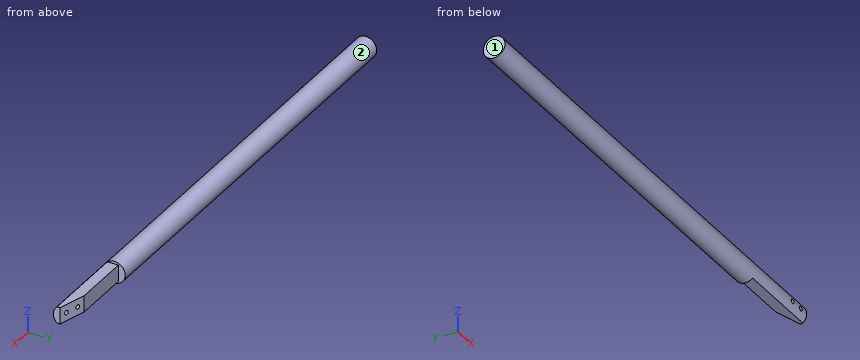
Autodesk Inventor part; units mm, degrees
ref_plane "YZ Plane" through (0, 0, 0) normal (1, 0, 0) x (0, 1, 0)
ref_plane "XZ Plane" through (0, 0, 0) normal (0, 1, 0) x (-1, 0, 0)
ref_plane "XY Plane" through (0, 0, 0) normal (0, 0, 1) x (1, 0, 0)
sketch "Sketch1" plane through (0, 0, 0) normal (1, 0, 0) x (0, 1, 0)
  circle A0 centre (0, 0) radius 6.35
  dimension "d159" = 12.7
extrude "Extrusion1" add sketch "Sketch1" against normal blind 304.8
sketch "Sketch2" plane through (0, 0, 0) normal (1, 0, 0) x (0, 0, -1)
  arc A0 (5.9242, 2.286) -> (-5.9242, 2.286) centre (0, 0) ccw
  circle A1 centre (0, 0) radius 6.35
  line L0 (-5.9242, 2.286) -> (5.9242, 2.286)
  dimension "d111" = 4.064
extrude "Extrusion2" cut sketch "Sketch2" against normal blind 50.8 contours L0 A0
sketch "Sketch5" plane through (0, 2.286, 5.9242) normal (0, 1, 0) x (1, 0, 0)
  line L0 (0, 5.9242) -> (0, 10.7502)
  line L1 (0, 11.8485) -> (0, 0)
  line L2 (0, 10.7502) -> (-50.8, 10.7502)
  line L3 (-50.8, 11.8485) -> (-50.8, 0)
  line L4 (0, 5.9242) -> (0, 1.0982)
  line L5 (0, 1.0982) -> (-50.8, 1.0982)
  line L6 (-50.8, 1.0982) -> (-50.8, -4.826)
  line L7 (-50.8, -4.826) -> (10.2611, -4.826)
  line L8 (10.2611, -4.826) -> (0, 1.0982)
  line L9 (-50.8, 10.7502) -> (-50.8, 16.6745)
  line L10 (-50.8, 16.6745) -> (10.2611, 16.6745)
  line L11 (0, 10.7502) -> (10.2611, 16.6745)
  line L12 (-50.8, 11.8485) -> (0, 11.8485)
  dimension "d20" = 4.826
  dimension "d21" = 4.826
  dimension "d160" = 4.826
extrude "Extrusion3" cut sketch "Sketch5" against normal blind 25.4 contours L2 L3 L12 L1 | L1 L12 L9 L10 L11 | L8 L7 L6 L3 L5
sketch "Sketch18" plane through (-50.8, 2.286, 4.826) normal (0, 0, 1) x (1, 0, 0)
  line L0 (34.4586, 0) -> (50.8, -4.6858)
  line L1 (0, 0) -> (50.8, 0)
  line L2 (34.4586, 0) -> (50.8, 0)
  line L3 (50.8, 0) -> (50.8, -4.6858)
  dimension "d144" = 17
  dimension "d161" = 74
extrude "Extrusion9" cut sketch "Sketch18" against normal blind 25.4
sketch "Sketch19" plane through (-16.3414, 2.286, 4.826) normal (0.2756374, 0.9612617, 0) x (0.9612617, -0.2756374, 0)
  circle A0 centre (12.4695, 4.826) radius 1.5875
  circle A1 centre (4.532, 4.826) radius 1.5875
  line L0 (14.057, 4.826) -> (17, 4.826)
  line L1 (17, 9.652) -> (17, 0)
  line L2 (14.057, 4.826) -> (4.532, 4.826) construction
  dimension "d148" = 3.175
  dimension "d149" = 3.175
  dimension "d151" = 7.9375
  dimension "d162" = 2.943
hole "Hole9" at (-11.985, 1.0368, 0) at (-4.355, -1.1511, 0) direction (-0.2756374, -0.9612617, 0) diameter 2.4867 end through all
equation "\"d160\" = d20"
properties part number "rat_headbarAngled" material "Stainless Steel"
Check sheet for the modelled part. Datum: model origin and axes. Units: mm. Face numbers are marked on the shaded views. Give positions to 0.01 mm unless a question says otherwise; leave off trailing zeros. Order: outer loops, then holes, each group sorted by start corner. A loop starts at its lowest first (then second) coordinate and runs counter-clockwise, first axis right, second up. Notation, with made-up numbers: M 77.5,0 L 86.5,0 A14 ccw 86.5,9 Z; hole C 36,22.5 d10. An arc over 180 degrees is marked long. Answer as CSV lines item,"result". Start each with the question number.
Item 1: Thickness scan on line 1 (X direction, y = 3.25, z = 1.75); line 2 (Z direction, x = -53, y = 0.5); line 3 (Z direction, x = -33, y = -2). Record the ranges inside material, lowest first. Write a range as [from, to].
Item 2: Gauge pin test, flat ends, axial feed: P1, Ø3, axis at x = -25, y = -1, coming from the -Z side; P2, Ø4, axis at x = -242.5, z = 4.5, coming from the +Y side; P3, Ø6, axis at x = -87, y = -4, coming from the +Z side. Record the tip position at first contact, or that the pin passes through.
Item 3: Mould release check, pull along Z, two halves, no side actions. Record for the marked faces 1 and 2: +Z half, -Z half, draft (parallel to the pull), parting line (faces both ways), or undercut.
Item 4: Cross-section at A-A on x = -258. Enter the section's corners in (y, z).
Established:
1,line 1,"x = [-304.8, -50.8]"
1,line 2,"z = [-6.33, 6.33]"
1,line 3,"z = [-4.83, 4.83]"
2,P1,"stops at z = -4.83"
2,P2,"stops at y = 5.84"
2,P3,"stops at z = 6.27"
3,face 1,"draft"
3,face 2,"parting line"
4,outline,"C 0,0 d12.7"
